Here's how the part is built. I have some questions about the finished solid (model axes, mm). A direction names the side the tool comes from. Round coordinates to 2 decimals unless told otherwise and drop trailing zeros. Order: outer loops, then holes, each group sorted by start corner. A loop starts at its lowest first (then second) coordinate and runs counter-clockwise, first axis right, second up. Notation, with made-up numbers: (84.25, 21) -> (103.25, 21) arc R4 ccw to (103.25, 26) -> close; hole circle Ø9 at (5.5, 40). An arc over 180 degrees is marked (long way). One line per item, written item: value.
Autodesk Inventor part; units mm, degrees
ref_plane "YZ Plane" through (0, 0, 0) normal (1, 0, 0) x (0, 1, 0)
ref_plane "XZ Plane" through (0, 0, 0) normal (0, 1, 0) x (-1, 0, 0)
ref_plane "XY Plane" through (0, 0, 0) normal (0, 0, 1) x (1, 0, 0)
sketch "Sketch1" plane through (0, 0, 0) normal (0, 1, 0) x (-1, 0, 0)
  circle A0 centre (0, 0) radius 39.5
  circle A1 centre (0, 0) radius 10
  circle A2 centre (0, 0) radius 29
  circle A3 centre (29, 0) radius 2.75
  circle A4 centre (0, 29) radius 2.75
  circle A5 centre (-29, 0) radius 2.75
  circle A6 centre (0, -29) radius 2.75
  dimension "d2" = 58
  dimension "d0" = 79
  dimension "d1" = 20
  dimension "d3" = 5.5
  dimension "d6" = 360
extrude "Extrusion1" add sketch "Sketch1" along normal blind 10 contours A0 | A1 | A3 A2 A6 A5 A4
sketch "Sketch3" plane through (0, 10, 0) normal (0, 1, 0) x (1, 0, 0)
  line L0 (-34.5, 50.157) -> (-34.5, -49.8555)
  circle A0 centre (0, 0) radius 39.5
  point P0 (-34.5, -19.2354)
  point P1 (-34.5, 19.2354)
  dimension "d18" = 5
extrude "Extrusion3" cut sketch "Sketch3" along normal through all both and the other way through all contours L0 A0 picked at (-35.5583, 3.956)
sketch "Sketch4" plane through (0, 0, 0) normal (0, -1, 0) x (1, 0, 0)
  circle A0 centre (0, 0) radius 10.16
  dimension "d21" = 20.32
extrude "Extrusion4" cut sketch "Sketch4" against normal blind 3
sketch "Sketch5" plane through (0, 0, 0) normal (0, -1, 0) x (1, 0, 0)
  arc A0 (-34.5, -19.2354) -> (-34.5, 19.2354) centre (0, 0) ccw
  line L0 (-34.5, 19.2354) -> (-34.5, -19.2354)
  arc A1 (-32.2183, -19.1893) -> (-32.2183, 19.1893) centre (0, 0) ccw
  circle A2 centre (-29, 0) radius 2.75
  arc A3 (-34.9211, 4.6034) -> (-34.9211, -4.6034) centre (-29, 0) ccw
  arc A4 (-33.125, 4.3571) -> (-33.125, -4.3571) centre (-29, 0) ccw
  line L1 (-32.5, -18.1659) -> (-32.5, -5.8095)
  line L2 (-32.5, 5.8095) -> (-32.5, 18.1659)
  line L3 (-34.5, 19.2354) -> (-34.5, 5.831)
  line L4 (-34.5, -5.831) -> (-34.5, -19.2354)
  arc A5 (-32.2183, 19.1893) -> (-32.5, 18.1659) centre (-30.5, 18.1659) ccw
  arc A6 (-32.5, -18.1659) -> (-32.2183, -19.1893) centre (-30.5, -18.1659) ccw
  arc A7 (-33.125, 4.3571) -> (-32.5, 5.8095) centre (-34.5, 5.8095) ccw
  arc A8 (-32.5, -5.8095) -> (-33.125, -4.3571) centre (-34.5, -5.8095) ccw
  arc A9 (-34.5, -5.831) -> (-34.9211, -4.6034) centre (-36.5, -5.831) ccw
  arc A10 (-34.9211, 4.6034) -> (-34.5, 5.831) centre (-36.5, 5.831) ccw
  point P0 (-32.5, 18.7083)
  point P1 (-32.5, -18.7083)
  point P2 (-32.5, -4.8734)
  point P3 (-32.5, 4.8734)
  point P4 (-34.5, -5.099)
  point P5 (-34.5, 5.099)
  point P6 (-34.5, 5.831)
  point P7 (-34.5, -5.831)
  dimension "d24" = 2
  dimension "d25" = 1.5
  dimension "d26" = 2
  dimension "d27" = 2
  dimension "d32" = 7.5
extrude "Extrusion5" add sketch "Sketch5" along normal blind 25.4 contours L0 A4 A8 L1 A6 A1 A5 L2 A7 A0 | A9 A3 A10 L0 A4
sketch "Sketch6" plane through (-34.5, 10, -19.2354) normal (-1, 0, 0) x (0, 0, 1)
  circle A0 centre (29.3954, -15.875) radius 4.2498
  point P0 (19.2354, -10)
extrude "Extrusion6" cut sketch "Sketch6" against normal through all
properties part number "PZT cell"
Q1. For P1, Ø9, axis at x = 0, z = 29, coming from the -Y side; P2, Ø10, axis at y = -5.875, z = 10.16, coming from the -X side; P3, Ø2, axis at y = 6, z = 26, coming from the +X side, each with a flat end and sliding along its axis, tell me the tip position at first contact or that it passes through.
Answers:
P1: y = 0
P2: x = -34.62
P3: x = 30.58
Q2. I want a section at D-D on y = -9. Write out the boundary of the cut face in (x, z) (1 decimal).
Answers:
outline: (-34.9, -4.6) arc R2 cw to (-34.5, -5.8) -> (-34.5, -19.2) arc R39.5 ccw to (38.8, 7.3) -> (36.8, 7.3) arc R37.5 cw to (-32.2, -19.2) arc R2 cw to (-32.5, -18.2) -> (-32.5, -5.8) arc R2 ccw to (-33.1, -4.4) arc R6 cw to (-33.1, 4.4) arc R2 ccw to (-32.5, 5.8) -> (-32.5, 7.3) -> (-34.5, 7.3) -> (-34.5, 5.8) arc R2 cw to (-34.9, 4.6) arc R7.5 ccw to start; (-34.5, 13) -> (-32.5, 13) -> (-32.5, 18.2) arc R2 cw to (-32.2, 19.2) arc R37.5 cw to (35.2, 13) -> (37.3, 13) arc R39.5 ccw to (-34.5, 19.2) -> close
Q3. If we mould it in two halves opening along X, with no side actions, what happens to faces 1 (the face through (31.747, 4.93, -0.121)), 2 (the face through (-35, -13, 0)), 3 (the face through (-36.5, -12.5, -0.1)), 4 (the face through (-33.514, -4.598, 14.214))? For each: pulls with the +X half, pulls with the -X half, needs draft (parallel to the pull), parting line crosses it, or undercut.
Answers:
face 1: undercut
face 2: undercut
face 3: pulls with the -X half
face 4: needs draft
Q4. Which directions (+Z, -Z, +X, -X, +Y, -Y) give clear straight access to the entire face, cutting with the end or side of a thin tool? Please do faces 5 (the face through (-6, 0, 9)), 6 (the face through (-35.3, 0, 0.1)), 7 (the face through (-26.253, 4.93, -0.121)).
Answers:
face 5: -Y
face 6: +Z, -Z, -X, +Y
face 7: +Y, -Y
Q5. I want a section at C-C on z = 30.5. Write out the boundary of the cut face in (x, y).
Answers:
outline: (-25.1, -25.4) -> (-21.82, -25.4) -> (-21.82, 0) -> (-2.3, 0) -> (-2.3, 10) -> (-25.1, 10) -> close; (2.3, 0) -> (21.82, 0) -> (21.82, -25.4) -> (25.1, -25.4) -> (25.1, 10) -> (2.3, 10) -> close
Q6. I need wall thicknesses on line 1 along Z through (x, y) = (0, 4.75); line 2 along Z through (x, y) = (0, 1.6); line 3 along Y through (x, z) = (-33, 10). Which ranges of each line are inside material? Lowest first, please.
Answers:
line 1: -39.5 to -31.75, -26.25 to 26.25, 31.75 to 39.5
line 2: -39.5 to -31.75, -26.25 to -10.16, 10.16 to 26.25, 31.75 to 39.5
line 3: -25.4 to -10.12, -1.63 to 10
Q7. I want a section at A-A on z = 0. Write out the boundary of the cut face in (x, y), then the cut area to 3 significant figures.
Answers:
outline: (-36.5, -25.4) -> (-35, -25.4) -> (-35, 0) -> (-36.5, 0) -> close; (-34.5, 0) -> (-31.75, 0) -> (-31.75, 10) -> (-34.5, 10) -> close; (-26.25, 0) -> (-10.16, 0) -> (-10.16, 3) -> (10.16, 3) -> (10.16, 0) -> (26.25, 0) -> (26.25, 10) -> (-26.25, 10) -> close; (31.75, 0) -> (37.5, 0) -> (37.5, -25.4) -> (39.5, -25.4) -> (39.5, 10) -> (31.75, 10) -> close
area: 658 mm2
Q8. I want a section at B-B on x = 0. Write out the boundary of the cut face in (y, z).
Answers:
outline: (-25.4, -39.5) -> (10, -39.5) -> (10, -31.75) -> (0, -31.75) -> (0, -37.5) -> (-25.4, -37.5) -> close; (-25.4, 37.5) -> (0, 37.5) -> (0, 31.75) -> (10, 31.75) -> (10, 39.5) -> (-25.4, 39.5) -> close; (0, -26.25) -> (10, -26.25) -> (10, 26.25) -> (0, 26.25) -> (0, 10.16) -> (3, 10.16) -> (3, -10.16) -> (0, -10.16) -> close
